Part model, mm, in its own coordinate system. Round coordinates to 2 decimals unless told otherwise and drop trailing zeros. Loops run counter-clockwise (first coordinate to the right, second up) from the corner with the lowest first, then second, coordinate; pieces in that order, holes last. Notation, with made-up numbers: M 39,-31 L 70,-31 A18 ccw 70,-19 Z; hole C 49.5,26 d6. An arc over 180 degrees is marked long. Put each result on its own line as item: value. Start each with the question number.
Autodesk Inventor part; units mm, degrees
ref_plane "YZ Plane" through (0, 0, 0) normal (1, 0, 0) x (0, 1, 0)
ref_plane "XZ Plane" through (0, 0, 0) normal (0, 1, 0) x (-1, 0, 0)
ref_plane "XY Plane" through (0, 0, 0) normal (0, 0, 1) x (1, 0, 0)
sketch "スケッチ1" plane through (0, 0, 0) normal (1, 0, 0) x (0, 1, 0)
  line L0 (68.2079, 642.9582) -> (68.2079, -632.5418)
  circle A0 centre (78.2079, 14.9582) radius 1.5
  line L1 (88.2079, -632.5418) -> (68.2079, -632.5418)
  circle A1 centre (78.2079, -0.0418) radius 1.5
  circle A2 centre (78.2079, 14.9582) radius 1.5
  line L2 (68.2079, -5.0418) -> (88.2079, -5.0418)
  line L3 (68.2079, 19.9582) -> (88.2079, 19.9582)
  line L4 (87.2079, 642.9582) -> (87.2079, 7.4582)
  line L5 (68.2079, 19.9582) -> (68.2079, -5.0418)
  line L6 (88.2079, 19.9582) -> (88.2079, -5.0418)
  line L7 (88.2079, 642.9582) -> (88.2079, -632.5418)
  point P0 (0, 0)
  point P1 (-76.7921, 17.4582)
  point P2 (78.2079, -625.0418)
  dimension "d0" = 10
  dimension "d1" = 15
  dimension "d2" = 7.5
  dimension "d3" = 10
  dimension "d4" = 3
  dimension "d5" = 3
  dimension "d6" = 5
  dimension "d7" = 5
extrude "押し出し1" add sketch "スケッチ1" against normal blind 2 contours L3 L6 L2 L0
fillet "フィレット1" radius 2 4 edges at (-1, 88.2079, 19.9582) (-1, 68.2079, 19.9582) (-1, 88.2079, -5.0418) (-1, 68.2079, -5.0418)
properties part number "base_weel-v1-Plate-expand-2" material "アルミニウム 6061"
1. Cut at A-A, the plane z = 15.5. Give the cut face in (x, y), and give its area (3 significant figures).
2. Mould opens along Y. For faces 1 (the cylindrical face through (-1.01, 87.64, -4.44)), 2 (the cylindrical face through (-0.99, 79.64, 15.41)), 3 (the flat face through (-1, 78, -5.042)) say: released by +Y, released by -Y, zero draft, split by the parting line, or undercut.
3. Cut at B-B, the plane y = 77. Give the cut face in (x, z), and give its area (3 significant figures).
4. Cut at C-C, the plane z = -0.75. Give the cut face in (x, y), and give its area (3 significant figures).
5. Cut at D-D, the plane x = -1.4. Give the number of separate pieces and of enclosed holes in the cut face, and give its area (3 significant figures).
6. Wall check: L1, parallel to Z at x = -1.9, y = 79; L2, parallel to Y at x = -0.85, z = 0.25; L3, parallel to Y at x = -0.55, z = 15.5. Give the ranges that are in metal, low to high.
Results list:
1. outline: M -2,68.21 L 0,68.21 L 0,76.81 L -2,76.81 Z; M -2,79.61 L 0,79.61 L 0,88.21 L -2,88.21 Z
1. area: 34.4 mm^2
2. face 1: released by +Y
2. face 2: undercut
2. face 3: zero draft
3. outline: M -2,-5.04 L 0,-5.04 L 0,-0.93 L -2,-0.93 Z; M -2,0.85 L 0,0.85 L 0,14.07 L -2,14.07 Z; M -2,15.85 L 0,15.85 L 0,19.96 L -2,19.96 Z
3. area: 42.9 mm^2
4. outline: M -2,68.21 L 0,68.21 L 0,76.89 L -2,76.89 Z; M -2,79.53 L 0,79.53 L 0,88.21 L -2,88.21 Z
4. area: 34.7 mm^2
5. separate pieces: 1
5. enclosed holes: 2
5. area: 482 mm^2
6. L1: z = -5.04 to -1.32, 1.23 to 13.68, 16.23 to 19.96
6. L2: y = 68.21 to 76.74, 79.68 to 88.21
6. L3: y = 68.21 to 76.81, 79.61 to 88.21
